Could you check a few things on this model? Use its own coordinates, in mm. Face numbers are marked on the shaded views. A direction names the side the tool comes from. Coordinates: 2 decimals unless noted, no trailing zeros. Loops run counter-clockwise (first coordinate to the right, second up) from the corner with the lowest first, then second, coordinate; pieces in that order, holes last. Notation, with made-up numbers: (81.5, -36) - (133.5, -36) arc R31 ccw to (133.5, -7) - close; hole circle Ø1 at (86.25, 11.25). An arc over 180 degrees is marked (long way). One line per question, with ' | ' between items. Start each with the question number.
1. I want a section at B-B, the plane z = 17. Write out the boundary of the cut face in (x, y).
2. I want a section at A-A, the plane y = 19. Write out the boundary of the cut face in (x, z).
3. We'd pull the mould along X, two halves only. Please class the marked faces 1, 2 and 3: pulls with the +X half, pulls with the -X half, needs draft (parallel to the pull), parting line crosses it, or undercut.
4. I want a section at D-D, the plane z = 37. Write out the boundary of the cut face in (x, y), then the cut area to 3 significant figures.
5. I'm going to push flat-ended pins straight in: P1, Ø4, axis at y = 13.5, z = 36.5, coming from the -X side; P2, Ø6, axis at x = 32, z = 16.5, coming from the +Y side; P3, Ø9, axis at x = 38.5, y = 12, coming from the +Z side. Where does each tip first touch, or does it pass through?
6. Please list where these lines run through material, in increasing order: L1, parallel to X at y = 18, z = 7; L2, parallel to Y at x = 69, z = 3; L3, parallel to X at y = 57.5, z = 35.5. Write a range as [from, to].
7. Which directions (+Z, -Z, +X, -X, +Y, -Y) give clear straight access to the entire face, cutting with the end or side of a thin tool? Please do the marked faces 4, 5 and 6.
8. I want a section at C-C, the plane x = 41.5. Write out the boundary of the cut face in (y, z), then the cut area to 3 significant figures.
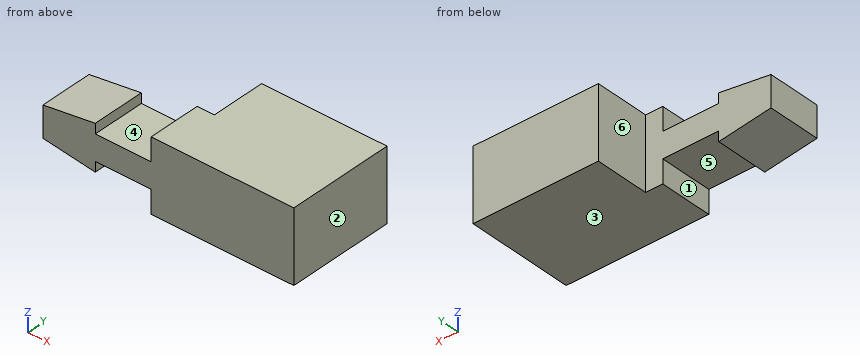
Autodesk Inventor part; units mm, degrees
ref_plane "YZ Plane" through (0, 0, 0) normal (1, 0, 0) x (0, 1, 0)
ref_plane "XZ Plane" through (0, 0, 0) normal (0, 1, 0) x (-1, 0, 0)
ref_plane "XY Plane" through (0, 0, 0) normal (0, 0, 1) x (1, 0, 0)
sketch "Boceto1" plane through (0, 0, 0) normal (0, 0, 1) x (1, 0, 0)
  line L0 (0, 0) -> (140, 0)
  line L1 (140, 0) -> (140, 60)
  line L2 (140, 60) -> (0, 60)
  line L3 (0, 60) -> (0, 0)
  dimension "d0" = 140
  dimension "d1" = 60
extrude "Extrusión1" add sketch "Boceto1" along normal blind 40
sketch "Boceto2" plane through (0, 60, 0) normal (0, 1, 0) x (1, 0, 0)
  line L0 (140, -40) -> (0, -40)
  line L1 (0, 0) -> (0, -40)
  line L2 (140, 0) -> (0, 0)
  line L3 (0, 0) -> (70, 0)
  line L4 (0, 0) -> (70, 0) construction
  line L5 (70, 0) -> (70, -40)
  line L6 (0, -40) -> (70, -40)
  point P0 (70, 0)
  dimension "d4" = 70
  dimension "d5" = 0
extrude "Extrusión2" cut sketch "Boceto2" against normal blind 30.4
sketch "Boceto3" plane through (0, 0, 0) normal (0, -1, 0) x (1, 0, 0)
  line L0 (0, 0) -> (140, 0)
  line L1 (0, 0) -> (0, 11.4)
  line L2 (0, 0) -> (0, 40)
  line L3 (0, 11.4) -> (0, 28.6) construction
  line L4 (0, 28.6) -> (0, 40)
  line L5 (0, 0) -> (29.2, 0)
  line L6 (29.2, 0) -> (29.2, 7.4) construction
  line L7 (0, 11.4) -> (29.2, 7.4)
  line L8 (29.2, 0) -> (29.2, 7.4)
  line L9 (29.2, 7.4) -> (29.2, 12.9)
  line L10 (29.2, 12.9) -> (60.4, 12.9)
  line L11 (29.2, 0) -> (60.4, 0)
  line L12 (60.4, 0) -> (60.4, 12.9)
  line L13 (0, 40) -> (140, 40)
  line L14 (0, 40) -> (60.4, 40)
  line L15 (60.4, 40) -> (60.4, 27.1)
  line L16 (60.4, 27.1) -> (29.2, 27.1)
  line L17 (60.4, 27.1) -> (91.6, 27.1) construction
  line L18 (29.2, 27.1) -> (29.2, 32.6)
  line L19 (29.2, 32.6) -> (0, 28.6)
  dimension "d8" = 11.4
  dimension "d9" = 17.2
  dimension "d10" = 29.2
  dimension "d11" = 7.4
  dimension "d12" = 5.5
  dimension "d13" = 31.2
  dimension "d14" = 12.9
  dimension "d15" = 60.4
  dimension "d16" = 31.2
  dimension "d17" = 180
  dimension "d18" = 5.5
extrude "Extrusión3" cut sketch "Boceto3" against normal blind 30
equation "\"d4\" = Largo_mitad"
equation "\"d12\" = Prof_corte"
equation "\"d18\" = Prof_corte"
equation "\"Largo_mitad\" = 70"
equation "\"Prof_corte\" = 5.5"
equation "\"Separacion_1\" = 11"
equation "\"Separacion_2\" = 7"
equation "\"Separacion_3\" = 12.5"
equation "\"Angulo_0\" = 0"
equation "\"Angulo_180\" = 180deg"
properties part number "Tenon_Macho_Parametrizado"
Results are:
1) outline: (0, 0) - (140, 0) - (140, 60) - (70, 60) - (70, 29.6) - (0, 29.6) - close
2) outline: (0, 11.4) - (29.2, 7.4) - (29.2, 12.9) - (60.4, 12.9) - (60.4, 0) - (140, 0) - (140, 40) - (60.4, 40) - (60.4, 27.1) - (29.2, 27.1) - (29.2, 32.6) - (0, 28.6) - close
3) face 1: undercut | face 2: pulls with the +X half | face 3: needs draft
4) outline: (60.4, 0) - (140, 0) - (140, 60) - (70, 60) - (70, 29.6) - (60.4, 29.6) - close | area: 4,480 mm2
5) P1: stops at x = 60.4 | P2: stops at y = 29.6 | P3: stops at z = 27.1
6) L1: x = [60.4, 140] | L2: y = [0, 29.6] | L3: x = [70, 140]
7) face 4: +Z, +Y, -Y | face 5: -Z, +Y, -Y | face 6: +Z, -Z, -X, +Y
8) outline: (0, 12.9) - (29.6, 12.9) - (29.6, 27.1) - (0, 27.1) - close | area: 420 mm2
